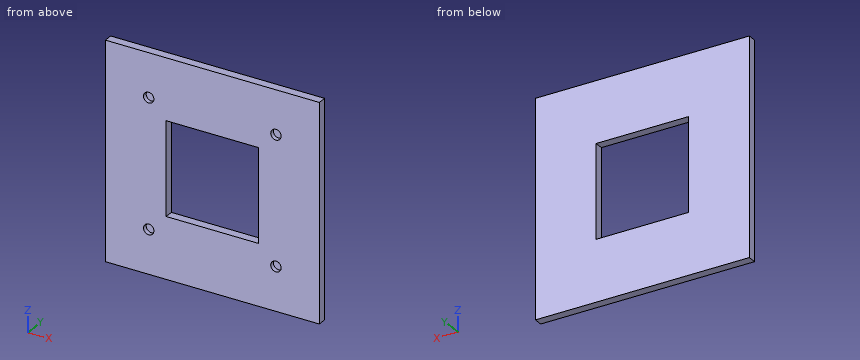
from build123d import *

# Parameters (mm, degrees)
SKETCH1_W           = 74
SKETCH1_H           = 74
SKETCH1_W_2         = 32
SKETCH1_H_2         = 32
BOSS_EXTRUDE1_DEPTH = 3
SKETCH3_R           = 1.8
CUT_EXTRUDE1_DEPTH  = 1.5


with BuildPart() as part:
    # Sketch1 → Boss-Extrude1 (new body)
    with BuildSketch(Plane(origin=(0, 0, 0), x_dir=(1, 0, 0), z_dir=(0, 1, 0))):
        Rectangle(SKETCH1_W, SKETCH1_H)
        Rectangle(SKETCH1_W_2, SKETCH1_H_2, mode=Mode.SUBTRACT)
    extrude(amount=BOSS_EXTRUDE1_DEPTH)

    # Sketch3 → Cut-Extrude1 (cut)
    with BuildSketch(Plane(origin=(0, 0, 0), x_dir=(1, 0, 0), z_dir=(0, 1, 0))):
        with Locations((-22, 22)):
            Circle(SKETCH3_R)
        with Locations((22, 22)):
            Circle(SKETCH3_R)
        with Locations((22, -22)):
            Circle(SKETCH3_R)
        with Locations((-22, -22)):
            Circle(SKETCH3_R)
    extrude(amount=CUT_EXTRUDE1_DEPTH, mode=Mode.SUBTRACT)


solid = part.part
Part model, mm, in its own coordinate system. Coordinates: 2 decimals unless noted, no trailing zeros. Order: outer loops, then holes, each group sorted by start corner. A loop starts at its lowest first (then second) coordinate and runs counter-clockwise, first axis right, second up.
(1) Pin check, flat tip, straight feed: pin 1 Ø1.8 at (x, z) = (-22.5, -22) entering from -Y. Stop position of the tip, or through.
Check sheet entries:
pin 1: stops at y = 1.5
(2) Slice it at D-D, the plane x = -22. Write the cut outline in (y, z), and give its area (3 significant figures).
Check sheet entries:
outline: (0, -37) - (3, -37) - (3, 37) - (0, 37) - (0, 23.8) - (1.5, 23.8) - (1.5, 20.2) - (0, 20.2) - (0, -20.2) - (1.5, -20.2) - (1.5, -23.8) - (0, -23.8) - close
area: 211 mm2
(3) Probe L1, parallel to X at y = 0.6, z = 22; L2, parallel to Z at x = 1, y = 0.4. List the from-to ranges inside material, lowest first.
Check sheet entries:
L1: x = -37 to -23.8, -20.2 to 20.2, 23.8 to 37
L2: z = -37 to -16, 16 to 37
(4) Slice it at A-A, the plane y = 0.75. Write the cut outline in (x, z), and give its area (3 significant figures).
Check sheet entries:
outline: (-37, -37) - (37, -37) - (37, 37) - (-37, 37) - close; hole circle Ø3.6 at (-22, -22); hole circle Ø3.6 at (-22, 22); hole (-16, -16) - (16, -16) - (16, 16) - (-16, 16) - close; hole circle Ø3.6 at (22, -22); hole circle Ø3.6 at (22, 22)
area: 4,410 mm2
(5) Slice it at C-C, the plane z = 9. Write the cut outline in (x, y), and give its area (3 significant figures).
Check sheet entries:
outline: (-37, 0) - (-16, 0) - (-16, 3) - (-37, 3) - close; (16, 0) - (37, 0) - (37, 3) - (16, 3) - close
area: 126 mm2
(6) Slice it at B-B, the plane x = -2.5. Write the cut outline in (y, z), and give its area (3 significant figures).
Check sheet entries:
outline: (0, -37) - (3, -37) - (3, -16) - (0, -16) - close; (0, 16) - (3, 16) - (3, 37) - (0, 37) - close
area: 126 mm2
